Source: CAD feature listing. Evaluate the final solid. Frame: model axes, mm. Round coordinates to 2 decimals unless told otherwise and drop trailing zeros. Order: outer loops, then holes, each group sorted by start corner. A loop starts at its lowest first (then second) coordinate and runs counter-clockwise, first axis right, second up. Notation, with made-up numbers: (47.5, 81.5) -> (62.5, 81.5) arc R20 cw to (62.5, 114.5) -> close; hole circle Ø10 at (88, -23). An arc over 180 degrees is marked (long way). Write item = value, one per line. Start each with the question number.
(1) Contact query for flat-ended pins moving along their axis: pin 1 Ø10 at (y, z) = (1.5, -14) entering from -X; pin 2 Ø1.5 at (y, z) = (-19.5, -4.5) entering from -X; pin 3 Ø5 at (y, z) = (-35.5, -12.5) entering from +X. Output: stop coordinate, or through.
(2) Draft query along Y for faces 1 (the face through (-12.3, -41.44, -2.17)), 2 (the face through (-19.864, -18.584, -12.395)), 3 (the face through (0, -31, -20)), 4 (the face through (14.477, -45.148, -11.264)). Return one class per face: released by +Y, released by -Y, zero draft, split by the parting line, or undercut.
(3) Cut plane A-A on x = 0. Return the cut outline in (y, z).
(4) Cut plane C-C on z = -4. Return the cut outline in (x, y), then the cut area to 3 significant figures.
(5) Ray query, line 1 (X direction, y = -43, z = -13.5); line 2 (Y direction, x = 0, z = -15); line 3 (X direction, y = -44.5, z = -14.5). Return the intervals inside material, ascending.
(6) Cut plane B-B on z = -14.25. Return the cut outline in (x, y).
from build123d import *

# Parameters (mm, degrees)
F1_DEPTH       = 20
F2_D           = 4.4
F2_CSINK_D     = 8.96
F2_CSINK_ANGLE = 90
F3_R           = 5
F4_D           = 7


# Not quite as in the source:
# - a feature names something its author has since deleted; it is built from what else it names


with BuildPart() as f1:
    # F0 (on Top) → F1 (new body)
    with BuildSketch(Plane.XY):
        with BuildLine():
            Line((-9.7258236175, -61), (9.7258236175, -61))
            ThreePointArc((9.7258236175, -61), (22.2857339512, -54.9120458236), (25.2876244635, -41.2810815511))
            Line((25.2876244635, -41.2810815511), (14.5891882931, 3.4864860458))
            ThreePointArc((14.5891882931, 3.4864860458), (0, 15), (-14.5891882931, 3.4864860458))
            Line((-14.5891882931, 3.4864860458), (-25.2876244635, -41.2810815511))
            ThreePointArc((-25.2876244635, -41.2810815511), (-22.2857339512, -54.9120458236), (-9.7258236175, -61))
        make_face()
    extrude(amount=-F1_DEPTH)

    # F2 (through all)
    with Locations(Plane.XY):
        with Locations((-14, -43), (14, -43)):
            CounterSinkHole(F2_D / 2, F2_CSINK_D / 2, counter_sink_angle=F2_CSINK_ANGLE)

    # F3
    f3_edges = [f1.edges().sort_by_distance(p)[0] for p in [
        (0, -61, 0),
        (-19.938406, -18.897298, 0),
        (19.938406, -18.897298, 0),
    ]]
    fillet(f3_edges, radius=F3_R)

    # F4 (through all)
    with Locations(Plane.XY):
        with Locations((0, 0)):
            Hole(F4_D / 2)


solid = f1.part
Evaluation:
q1.pin_1 = -16.26
q1.pin_2 = -20.25
q1.pin_3 = 24.5
q2.face_1 = undercut
q2.face_2 = released by +Y
q2.face_3 = zero draft
q2.face_4 = undercut
q3.outline = (-61, -20) -> (-3.5, -20) -> (-3.5, 0) -> (-56, 0) arc R5 ccw to (-61, -5) -> close; (3.5, -20) -> (15, -20) -> (15, -5) arc R5 ccw to (10, 0) -> (3.5, 0) -> close
q4.outline = (-25.19, -41.3) arc R15.9 ccw to (-9.73, -60.9) -> (9.73, -60.9) arc R15.9 ccw to (25.19, -41.3) -> (14.49, 3.46) arc R14.9 ccw to (-14.49, 3.46) -> close; hole circle Ø4.4 at (-14, -43); hole circle Ø7 at (0, 0); hole circle Ø4.4 at (14, -43)
q4.area = 2,850 mm^2
q5.line_1 = -25.6 to -16.2, -11.8 to 11.8, 16.2 to 25.6
q5.line_2 = -61 to -3.5, 3.5 to 15
q5.line_3 = -25.72 to -15.61, -12.39 to 12.39, 15.61 to 25.72
q6.outline = (-25.29, -41.28) arc R16 ccw to (-9.73, -61) -> (9.73, -61) arc R16 ccw to (25.29, -41.28) -> (14.59, 3.49) arc R15 ccw to (-14.59, 3.49) -> close; hole circle Ø4.4 at (-14, -43); hole circle Ø7 at (0, 0); hole circle Ø4.4 at (14, -43)
